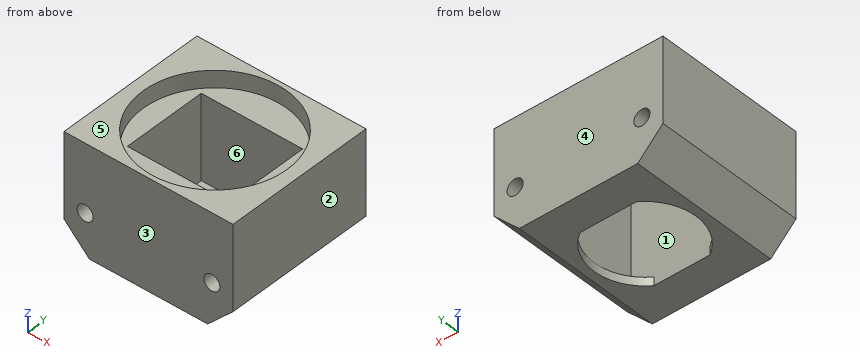
Autodesk Inventor part; units mm, degrees
ref_plane "YZ Plane" through (0, 0, 0) normal (1, 0, 0) x (0, 1, 0)
ref_plane "XZ Plane" through (0, 0, 0) normal (0, 1, 0) x (-1, 0, 0)
ref_plane "XY Plane" through (0, 0, 0) normal (0, 0, 1) x (1, 0, 0)
sketch "Sketch1" plane through (0, 0, 0) normal (0, 0, 1) x (1, 0, 0)
  line L0 (0, 0) -> (20, 0)
  line L1 (20, 0) -> (20, 18)
  line L2 (20, 18) -> (0, 18)
  line L3 (0, 18) -> (0, 0)
  dimension "d0" = 20
  dimension "d1" = 18
extrude "body" add sketch "Sketch1" along normal blind 13
sketch "Sketch2" plane through (0, 18, 0) normal (0, 1, 0) x (1, 0, 0)
  line L0 (20, 0) -> (0, 0)
  point P0 (2.5, -5)
  point P1 (17.5, -5)
  dimension "d4" = 2.5
  dimension "d5" = 2.5
  dimension "d6" = 5
  dimension "d7" = 5
hole "top mount" at (2.5, 18, 5) at (17.5, 18, 5) direction (0, -1, 0) diameter 1.9 depth 4
sketch "Sketch3" plane through (0, 0, 0) normal (0, -1, 0) x (1, 0, 0)
  line L0 (0, 0) -> (20, 0)
  point P0 (17.5, 5)
  point P1 (2.5, 5)
  dimension "d15" = 5
  dimension "d16" = 5
  dimension "d17" = 2.5
  dimension "d18" = 2.5
hole "bottom mount" at (17.5, 0, 5) at (2.5, 0, 5) direction (0, 1, 0) diameter 1.9 depth 4
sketch "Sketch4" plane through (0, 0, 13) normal (0, 0, 1) x (1, 0, 0)
  point P0 (0, 0)
  point P1 (0, 18)
  point P2 (10, 9)
  dimension "d26" = 10
  dimension "d27" = 9
hole "spool" at (10, 9, 13) direction (0, 0, -1) diameter 17 depth 2
sketch "Sketch5" plane through (0, 0, 13) normal (0, 0, 1) x (1, 0, 0)
  line L0 (4, 4) -> (16, 4)
  line L1 (16, 4) -> (16, 14)
  line L2 (16, 14) -> (4, 14)
  line L3 (4, 14) -> (4, 4)
  line L4 (4, 4) -> (16, 14) construction
  line L5 (16, 4) -> (4, 14) construction
  point P0 (0, 0)
  point P1 (10, 9)
  dimension "d35" = 12
  dimension "d36" = 10
extrude "gearbox pocket" cut sketch "Sketch5" against normal blind 12
sketch "Sketch6" plane through (0, 0, 1) normal (0, 0, 1) x (1, 0, 0)
  line L0 (13.3166, 4) -> (6.6834, 4)
  line L1 (6.6834, 4) -> (6.6834, 14)
  line L2 (6.6834, 14) -> (13.3166, 14)
  line L3 (13.3166, 14) -> (13.3166, 4)
  line L4 (13.3166, 4) -> (6.6834, 14) construction
  line L5 (6.6834, 4) -> (13.3166, 14) construction
  arc A0 (13.3166, 4) -> (13.3166, 14) centre (10, 9) ccw
  arc A1 (6.6834, 4) -> (13.3166, 4) centre (10, 9) ccw construction
  arc A2 (13.3166, 14) -> (6.6834, 14) centre (10, 9) ccw construction
  arc A3 (6.6834, 14) -> (6.6834, 4) centre (10, 9) ccw
  dimension "d46" = 12
  dimension "d47" = 10
extrude "Extrusion3" cut sketch "Sketch6" against normal through all
chamfer "Chamfer1" distance 3 angle 45 2 edges at (0, 9, 0) (20, 9, 0)
properties part number "drive R"
CAD build for the part. Positions are in the model's coordinates, mm. Face numbers are marked on the shaded views. A direction names the side the tool comes from. Round coordinates to 2 decimals unless told otherwise and drop trailing zeros. Loops run counter-clockwise (first coordinate to the right, second up) from the corner with the lowest first, then second, coordinate; pieces in that order, holes last. Notation, with made-up numbers: M -4,2.5 L 3,2.5 A18 ccw 3,20.5 Z; hole C -26,-32 d6. An arc over 180 degrees is marked long. Use a Markdown table: item, result. Add a question column.
(1) Drill centre lines: line 1 (X direction, y = 15.15, z = 5); line 2 (Y direction, x = 4.5, z = 5); line 3 (Z direction, x = 17.5, y = 16.05). Where is each one in solid material? Low to high.
(2) Which spindle directions (+Z, -Z, +X, -X, +Y, -Y) get a long thin tool onto all of the face, cutting with end or side? Do the marked faces 5 and 6. Say none if no direction does.
(3) Cut at C-C (z = 11.5). Give the cut face in (x, y).
(4) Flat gauge pins, fed straight in: pin 1 (1.5 mm diameter, centred on x = 17.5, z = 5, fed in from -Y); pin 2 (2 mm diameter, centred on x = 15.5, y = 9, fed in from +Z). Where does each tip first touch, or does it go through?
(5) Cut at D-D (y = 2.5). Give the cut face in (x, z).
(6) Pull direction Y, two halves, no side cores. Call the marked faces 1, 2, 3 and 4: +Y half, -Y half, draft (parallel to the pull), parting line (faces both ways), or undercut.
(7) Cut at B-B (x = 10). Give the cut face in (y, z), and give its area (3 significant figures).
Geometry says:
| question | item | result |
|---|---|---|
| 1 | line 1 | x = 0 to 1.55, 3.45 to 16.55, 18.45 to 20 |
| 1 | line 2 | y = 0 to 4, 14 to 18 |
| 1 | line 3 | z = 0.5 to 4.05, 5.95 to 13 |
| 2 | face 5 | +Z, +X, -X, +Y, -Y |
| 2 | face 6 | +Z |
| 3 | outline | M 0,0 L 20,0 L 20,18 L 0,18 Z; hole C 10,9 d17 |
| 4 | pin 1 | stops at y = 4 |
| 4 | pin 2 | stops at z = 11 |
| 5 | outline | M 0,3 L 3,0 L 17,0 L 20,3 L 20,13 L 15.48,13 L 15.48,11 L 4.52,11 L 4.52,13 L 0,13 Z; hole C 2.5,5 d1.9; hole C 17.5,5 d1.9 |
| 6 | face 1 | undercut |
| 6 | face 2 | draft |
| 6 | face 3 | -Y half |
| 6 | face 4 | +Y half |
| 7 | outline | M 0,0 L 4,0 L 4,11 L 0.5,11 L 0.5,13 L 0,13 Z; M 14,0 L 18,0 L 18,13 L 17.5,13 L 17.5,11 L 14,11 Z |
| 7 | area | 90.0 mm² |
